Verification items for this drawing (mm, ordinates from the low corner). A direction names the side the tool comes from. Give positions to 0.01 mm unless a question says otherwise; leave off trailing zeros. Loops run counter-clockwise (first coordinate to the right, second up) from the corner with the lowest first, then second, coordinate; pieces in that order, holes last. Notation, with made-up numbers: (48.5, 78.5) -> (107.5, 78.5) arc R23 ccw to (107.5, 111.5) -> close; hole circle Ø1 at (8.5, 33.5). An arc over 180 degrees is marked (long way). Write each question's results on one line, items separated by ' | '. Start each with the question number.
Item 1: Cross-section at C-C on x = 15. Enter the section's corners in (y, z).
Item 2: Cross-section at D-D on z = 8.75. Enter the section's corners in (x, y).
Item 3: Access from +Z, -Z, +X, -X, +Y, -Y to the whole of each face (thin tool, end or side, straight path). Record for the marked faces 1 and 2.
Item 4: Scan lines: line 1 along Y through (x, z) = (15.5, 12.5); line 2 along Y through (x, z) = (23, 15.25); line 3 along X through (y, z) = (2.25, 7.75). Record each from-to range of solid material in increasing order.
Item 5: Gauge pin test, flat ends, axial feed: pin 1 Ø0.5 at (y, z) = (2.5, 8.5) entering from -X; pin 2 Ø1.1 at (x, y) = (28.5, 3.5) entering from +Z; pin 3 Ø0.8 at (y, z) = (3.5, 9) entering from -X. Record the tip position at first contact, or that the pin passes through.
Item 6: Cross-section at B-B on z = 17.75. Enter the section's corners in (x, y).
Item 7: Cross-section at A-A on x = 23.5. Enter the section's corners in (y, z).
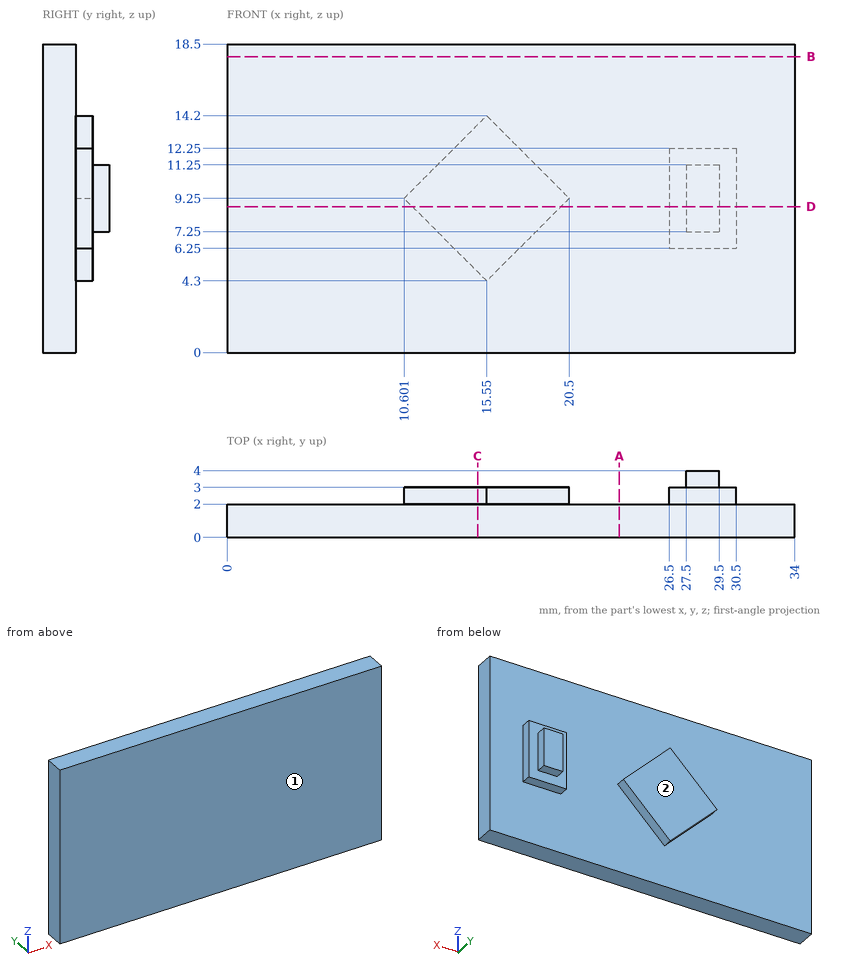
Answer sheet:
1) outline: (0, 0) -> (2, 0) -> (2, 4.85) -> (3, 4.85) -> (3, 13.65) -> (2, 13.65) -> (2, 18.5) -> (0, 18.5) -> close
2) outline: (0, 0) -> (34, 0) -> (34, 2) -> (30.5, 2) -> (30.5, 3) -> (29.5, 3) -> (29.5, 4) -> (27.5, 4) -> (27.5, 3) -> (26.5, 3) -> (26.5, 2) -> (20, 2) -> (20, 3) -> (11.1, 3) -> (11.1, 2) -> (0, 2) -> close
3) face 1: +Z, -Z, +X, -X, -Y | face 2: +Z, -Z, -X, +Y
4) line 1: y = 0 to 3 | line 2: y = 0 to 2 | line 3: x = 12.1 to 19, 26.5 to 30.5
5) pin 1: stops at x = 11.1 | pin 2: stops at z = 12.25 | pin 3: stops at x = 27.5
6) outline: (0, 0) -> (34, 0) -> (34, 2) -> (0, 2) -> close
7) outline: (0, 0) -> (2, 0) -> (2, 18.5) -> (0, 18.5) -> close
